Could you check a few things on this model? Use its own coordinates, in mm. A direction names the side the tool comes from. Round coordinates to 2 decimals unless told otherwise and drop trailing zeros. Order: outer loops, then holes, each group sorted by start corner. A loop starts at its lowest first (then second) coordinate and runs counter-clockwise, first axis right, second up.
```python
from build123d import *

# Parameters (mm, degrees)
CUT_EXTRUDE1_START = -1.62
CUT_EXTRUDE1_DEPTH = 1.62
SKETCH3_R          = 1.5
CUT_EXTRUDE2_DEPTH = 2


with BuildPart() as part:
    # Sketch1 → Revolve2 (revolve)
    with BuildSketch(Plane(origin=(0, 0, 0), x_dir=(0, 0, -1), z_dir=(1, 0, 0))):
        with BuildLine():
            Line((0, 0), (0, 2.555))
            Line((0, 2.555), (-74.8, 2.555))
            Line((-74.8, 2.555), (-74.8, 10.07))
            Line((-74.8, 10.07), (-79.91, 10.07))
            Line((-79.91, 10.07), (-271.422345798, 5.108285876))
            ThreePointArc((-271.422345798, 5.108285876), (-274.949807852, 3.566217392), (-276.4, 0))
            Line((-276.4, 0), (0, 0))
        make_face()
    revolve(axis=Axis((0, 0, 0), (0, 0, 1)))

    # Sketch2 → Cut-Extrude1 (cut)
    with BuildSketch(Plane(origin=(0, 0, 0), x_dir=(-1, 0, 0), z_dir=(0, 0, -1)).offset(CUT_EXTRUDE1_START)):
        with BuildLine():
            Line((0.81, -2.423205522), (0.81, 2.423205522))
            ThreePointArc((0.81, 2.423205522), (0, 2.555), (-0.81, 2.423205522))
            Line((-0.81, 2.423205522), (-0.81, -2.423205522))
            ThreePointArc((-0.81, -2.423205522), (0, -2.555), (0.81, -2.423205522))
        make_face()
    extrude(amount=CUT_EXTRUDE1_DEPTH, mode=Mode.SUBTRACT)

    # Sketch3 → Cut-Extrude2 (cut)
    with BuildSketch(Plane(origin=(0, 2.555, 0), x_dir=(1, 0, 0), z_dir=(0, 1, 0))):
        with Locations(Location((0, -70.175, 0), (0, 0, 270))):
            Circle(SKETCH3_R)
    extrude(amount=-CUT_EXTRUDE2_DEPTH, mode=Mode.SUBTRACT)


solid = part.part
```
Q1. For P1, Ø10, axis at y = -1.5, z = 230.5, coming from the +X side; P2, Ø5, axis at x = -0.5, y = -6, coming from the -Z side; P3, Ø8, axis at x = 8, z = 54, coming from the +Y side; P4, Ø0.9, axis at x = 0, z = 69.5, coming from the +Y side (3 decimals), each with a flat end and sliding along its axis, tell me the tip position at first contact or that it passes through.
Q2. I need wall thicknesses on L1, parallel to X at y = -2.5, z = 235; L2, parallel to Y at x = -6.75, z = 165.5; L3, parallel to X at y = 0.25, z = 146.5. Which ranges of each line are inside material? Lowest first, please.
Q3. Imagine slicing it at B-B, the plane z = 85.5. Please give me the cut outline in (x, y), then the cut area to 3 significant figures.
Q4. For faces 1 (the cylindrical face through (-9.984, -1.311, 77.391)), 2 (the flat face through (2, -2, 74.8)), 3 (the conical face through (7.375, -1.638, 177.007)), which set-ups out of +Z, -Z, +X, -X, +Y, -Y let a thin tool reach every point of the face, with its end or its side?
Q5. Imagine slicing it at A-A, the plane z = 23. Please give me the cut outline in (x, y) (3 decimals), then the cut area to 3 significant figures.
Filled in:
1. P1: stops at x = 6.29
1. P2: stops at z = 74.8
1. P3: passes through
1. P4: stops at y = 0.555
2. L1: x = -5.51 to 5.51
2. L2: y = -4.01 to 4.01
2. L3: x = -8.34 to 8.34
3. outline: circle Ø19.85 at (0, 0)
3. area: 309 mm2
4. face 1: +Z, -Z
4. face 2: -Z
4. face 3: +Z
5. outline: circle Ø5.11 at (0, 0)
5. area: 20.5 mm2
